Verification items for the finished model (mm, model axes). Give positions to 0.01 mm unless a question says otherwise; leave off trailing zeros. Write each loop counter-clockwise with the first axis right and the second up, starting at its lowest first coordinate (ties: lowest second). Pieces come first, ordered by that corner, then holes. Notation, with made-up numbers: (24, -19.5) - (49, -19.5) arc R19 cw to (49, 10.5) - close; hole circle Ø8 at (-2, 83.25). An arc over 180 degrees is marked (long way). Answer as a JSON object with one key per item and string values. Group by question number.
Item 1: Sectioned sample at D-D, the plane z = -15. Record the boundary of the cut face in (x, y) (3 decimals), and give its area (3 significant figures).
Item 2: Scan lines: line 1 along X through (y, z) = (2.8, -21.5); line 2 along Z through (x, y) = (136.5, 1.05); line 3 along Z through (x, y) = (187.5, 2.85). Record each from-to range of solid material in increasing order. Write a range as [from, to].
Item 3: Go/stop test with flat-tipped pins: pin 1 (1 mm diameter, centred on x = 292.5, y = 2, fed in from +Z); pin 2 (1 mm diameter, centred on x = 92, y = 1, fed in from +Z); pin 3 (1.6 mm diameter, centred on y = 1.5, z = -8.5, fed in from -X). Record where each tip stops, or that it passes through.
Item 4: Sectioned sample at A-A, the plane y = 2.25. Record the boundary of the cut face in (x, z).
Item 5: Sectioned sample at B-B, the plane z = -110.5. Record the boundary of the cut face in (x, y) (1 decimal).
Item 6: Sectioned sample at C-C, the plane x = 244.5. Record the boundary of the cut face in (y, z) (1 decimal), and give its area (3 significant figures).
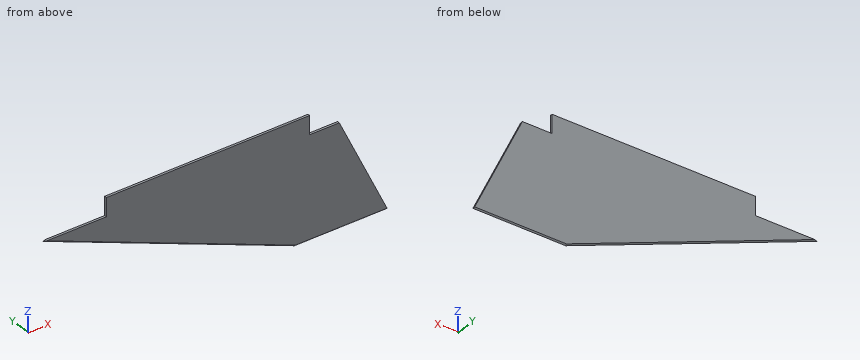
```python
from build123d import *

# Parameters (mm, degrees)
BOSS_EXTRUDE1_DEPTH = 3.175
CHAMFER1_SIZE       = 1.778


with BuildPart() as part:
    # Sketch1 → Boss-Extrude1 (new body)
    with BuildSketch(Plane(origin=(0, 0, 0), x_dir=(1, 0, 0), z_dir=(0, 1, 0))):
        Polygon((279.4, 25.4), (320.04, 25.4), (386.409633422, 165.1), (259.409633422, 165.1), (-86.36, 25.4), (0, 25.4), (0, 0), (279.4, 0), align=None)
    extrude(amount=BOSS_EXTRUDE1_DEPTH)

    # Chamfer1
    # the kernel refuses this chamfer: 1.778 mm, written as the material it takes off along each edge
    with BuildSketch(Plane(origin=(263.649137419, 3.175, -166.812870799), x_dir=(-0.01030013667007983, -0.9996219169112964, -0.02549373286050588), z_dir=(-0.9271838545667884, 0, 0.3746065934159097))) as chamfer1_piece_1:
        Polygon((CHAMFER1_SIZE * 0.999621916911, CHAMFER1_SIZE * 0.0274958766106), (-CHAMFER1_SIZE * 0.0274958766106, CHAMFER1_SIZE * 0.999621916911), (0, 0), align=None)
    extrude(amount=382.069467314, mode=Mode.SUBTRACT)
    with BuildSketch(Plane(origin=(263.649137419, 0, -166.812870799), x_dir=(-0.01030013667007983, 0.9996219169112964, -0.02549373286050588), z_dir=(-0.9271838545667884, 0, 0.3746065934159097))) as chamfer1_piece_2:
        Polygon((CHAMFER1_SIZE * 0.999621916911, -CHAMFER1_SIZE * 0.0274958766106), (-CHAMFER1_SIZE * 0.0274958766106, -CHAMFER1_SIZE * 0.999621916911), (0, 0), align=None)
    extrude(amount=382.069467314, mode=Mode.SUBTRACT)

    # Chamfer2
    # the kernel refuses this chamfer: 1.778 mm, written as the material it takes off along each edge
    with BuildSketch(Plane(origin=(397.383519069, 3.175, -165.1), x_dir=(0, 0.027495876610586497, 0.9996219169112968), z_dir=(-1, 0, 0))) as chamfer2_piece_1:
        with BuildLine():
            Line((1.828980941, 0), (-0.100540841, -1.826215437))
            Line((-0.100540841, -1.826215437), (-0.136087397, -1.825237684))
            ThreePointArc((-0.136087397, -1.825237684), (-0.060681766, -0.912821341), (-0.035546555, 0.000977753))
            Line((-0.035546555, 0.000977753), (0.000977753, 0.035546555))
            ThreePointArc((0.000977753, 0.035546555), (0.914776848, 0.010411345), (1.829958694, 0.035546555))
            Line((1.829958694, 0.035546555), (1.828980941, 0))
        make_face()
    extrude(amount=144.201458677, mode=Mode.SUBTRACT)
    with BuildSketch(Plane(origin=(397.383519069, 0, -165.1), x_dir=(0, -0.02749587661058638, 0.9996219169112968), z_dir=(-1, 0, 0))) as chamfer2_piece_2:
        with BuildLine():
            Line((1.828980941, 0), (-0.100540841, 1.826215437))
            Line((-0.100540841, 1.826215437), (-0.136087397, 1.825237684))
            ThreePointArc((-0.136087397, 1.825237684), (-0.060681766, 0.912821341), (-0.035546555, -0.000977753))
            Line((-0.035546555, -0.000977753), (0.000977753, -0.035546555))
            ThreePointArc((0.000977753, -0.035546555), (0.914776848, -0.010411345), (1.829958694, -0.035546555))
            Line((1.829958694, -0.035546555), (1.828980941, 0))
        make_face()
    extrude(amount=144.201458677, mode=Mode.SUBTRACT)


solid = part.part
```
Geometry check:
{
 "1": {"outline": "(0, 0) - (279.4, 0) - (279.4, 3.175) - (0, 3.175) - close", "area": "887 mm^2"},
 "2": {"line 1": "[0, 279.4]", "line 2": "[-114.66, 0]", "line 3": "[-134.48, 0]"},
 "3": {"pin 1": "z = -25.4", "pin 2": "z = 0", "pin 3": "x = 0"},
 "4": {"outline": "(-84.08, -25.4) - (259.58, -164.25) - (386, -164.25) - (320.04, -25.4) - (279.4, -25.4) - (279.4, 0) - (0, 0) - (0, -25.4) - close"},
 "5": {"outline": "(124.8, 1.6) - (129, 0) - (360.5, 0) - (360.5, 3.2) - (129, 3.2) - close"},
 "6": {"outline": "(0, -157.2) - (1.6, -158.9) - (3.2, -157.2) - (3.2, 0) - (0, 0) - close", "area": "502 mm^2"}
}
